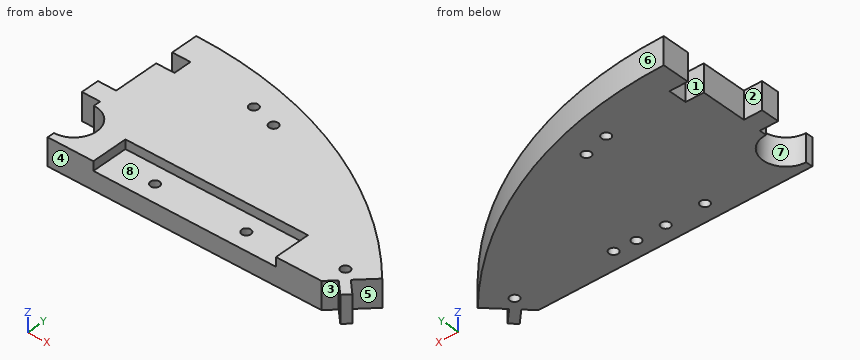
Autodesk Inventor part; units mm, degrees
ref_plane "YZ Plane" through (0, 0, 0) normal (1, 0, 0) x (0, 1, 0)
ref_plane "XZ Plane" through (0, 0, 0) normal (0, 1, 0) x (-1, 0, 0)
ref_plane "XY Plane" through (0, 0, 0) normal (0, 0, 1) x (1, 0, 0)
sketch "Sketch1" plane through (0, 0, 0) normal (0, 0, 1) x (1, 0, 0)
  circle A0 centre (0, -132.2876) radius 225 construction
  circle A1 centre (0, -132.2876) radius 200 construction
  line L0 (-225, -132.2876) -> (225, -132.2876) construction
  line L1 (150, -132.2876) -> (150, 35.4175) construction
  line L2 (175, -132.2876) -> (175, 9.1338) construction
  line L3 (0, 92.7124) -> (0, -357.2876) construction
  line L4 (150, 0) -> (0, 0)
  line L5 (0, 0) -> (0, 92.7124)
  line L6 (150, 0) -> (167.7086, 17.7086)
  line L7 (150, 0) -> (175.0437, 0) construction
  arc A2 (167.7086, 17.7086) -> (0, 92.7124) centre (0, -132.2876) ccw
  dimension "d0" = 450
  dimension "d1" = 25
  dimension "d2" = 75
  dimension "d3" = 25
  dimension "d4" = 45
extrude "Extrusion1" add sketch "Sketch1" along normal blind 15
sketch "Sketch2" plane through (0, 0, 15) normal (0, 0, 1) x (1, 0, 0)
  line L0 (10, 77.7124) -> (0, 77.7124)
  line L1 (0, 77.7124) -> (0, 67.7124)
  line L2 (0, 67.7124) -> (10, 67.7124)
  line L3 (10, 67.7124) -> (10, 77.7124)
  line L4 (0, 92.7124) -> (0, 0)
  line L5 (0, 0) -> (150, 0)
  line L6 (150, 0) -> (167.7086, 17.7086)
  arc A0 (167.7086, 17.7086) -> (0, 92.7124) centre (0, -132.2876) ccw
  line L7 (0, 92.7124) -> (0, 0)
  dimension "d7" = 10
  dimension "d8" = 10
  dimension "d21" = 15
extrude "Extrusion2" cut sketch "Sketch2" against normal blind 15 contours L3 L2 L1 L0
sketch "Sketch3" plane through (0, 0, 15) normal (0, 0, 1) x (1, 0, 0)
  line L0 (-10, 42.7124) -> (0, 42.7124)
  line L1 (0, 42.7124) -> (0, 32.7124)
  line L2 (0, 32.7124) -> (-10, 32.7124)
  line L3 (-10, 32.7124) -> (-10, 42.7124)
  line L4 (0, 0) -> (150, 0)
  line L5 (150, 0) -> (167.7086, 17.7086)
  arc A0 (167.7086, 17.7086) -> (0, 92.7124) centre (0, -132.2876) ccw
  line L6 (0, 67.7124) -> (0, 0)
  line L7 (0, 67.7124) -> (0, 0)
  line L8 (10, 67.7124) -> (0, 67.7124)
  line L9 (0, 92.7124) -> (0, 77.7124)
  line L10 (0, 77.7124) -> (10, 77.7124)
  line L11 (10, 77.7124) -> (10, 67.7124)
  dimension "d15" = 10
  dimension "d16" = 10
  dimension "d20" = 25
extrude "Extrusion3" add sketch "Sketch3" against normal blind 15 contours L0 L1 L2 L3
sketch "Sketch4" plane through (0, 0, 15) normal (0, 0, 1) x (1, 0, 0)
  line L0 (155, 5) -> (162.0711, -2.0711)
  line L1 (162.0711, -2.0711) -> (165.6066, 1.4645)
  line L2 (165.6066, 1.4645) -> (158.5355, 8.5355)
  line L3 (158.5355, 8.5355) -> (155, 5)
  line L4 (10, 67.7124) -> (0, 67.7124)
  line L5 (0, 67.7124) -> (0, 42.7124)
  line L6 (-10, 42.7124) -> (0, 42.7124)
  line L7 (-10, 32.7124) -> (-10, 42.7124)
  line L8 (0, 32.7124) -> (-10, 32.7124)
  line L9 (0, 32.7124) -> (0, 0)
  line L10 (0, 0) -> (150, 0)
  line L11 (150, 0) -> (167.7086, 17.7086)
  arc A0 (167.7086, 17.7086) -> (0, 92.7124) centre (0, -132.2876) ccw
  line L12 (0, 92.7124) -> (0, 77.7124)
  line L13 (0, 77.7124) -> (10, 77.7124)
  line L14 (10, 77.7124) -> (10, 67.7124)
  line L15 (150, 0) -> (167.7086, 17.7086)
  dimension "d22" = 10
  dimension "d23" = 5
  dimension "d24" = 5
extrude "Extrusion4" add sketch "Sketch4" against normal blind 15 contours L3 L2 L1 L0
sketch "Sketch5" plane through (0, 0, 15) normal (0, 0, 1) x (1, 0, 0)
  line L0 (10, 67.7124) -> (0, 67.7124) construction
  line L1 (0, 67.7124) -> (0, 42.7124) construction
  line L2 (-10, 42.7124) -> (0, 42.7124) construction
  line L3 (-10, 32.7124) -> (-10, 42.7124) construction
  line L4 (0, 32.7124) -> (-10, 32.7124) construction
  line L5 (0, 32.7124) -> (0, 0) construction
  line L6 (0, 0) -> (150, 0) construction
  line L7 (150, 0) -> (155, 5) construction
  line L8 (155, 5) -> (162.0711, -2.0711) construction
  line L9 (162.0711, -2.0711) -> (165.6066, 1.4645) construction
  line L10 (165.6066, 1.4645) -> (158.5355, 8.5355) construction
  line L11 (158.5355, 8.5355) -> (167.7086, 17.7086) construction
  arc A0 (167.7086, 17.7086) -> (0, 92.7124) centre (0, -132.2876) ccw construction
  line L12 (0, 92.7124) -> (0, 77.7124) construction
  line L13 (0, 77.7124) -> (10, 77.7124) construction
  line L14 (10, 77.7124) -> (10, 67.7124) construction
  circle A1 centre (0, -132.2876) radius 225 construction
  arc A2 (167.7086, 17.7086) -> (0, 92.7124) centre (0, -132.2876) ccw construction
  circle A3 centre (0, -132.2876) radius 210 construction
  circle A4 centre (50, 71.6732) radius 2.5
  circle A5 centre (64.4318, 67.5838) radius 2.5
  circle A6 centre (152.0028, 12.6094) radius 2.5
  dimension "d27" = 450
  dimension "d28" = 15
  dimension "d31" = 5
  dimension "d32" = 5
  dimension "d33" = 15
  dimension "d34" = 50
  dimension "d46" = 5
  dimension "d49" = 7.5
extrude "Extrusion5" cut sketch "Sketch5" against normal through all
thread "Thread1"
thread "Thread2"
thread "Thread4"
sketch "Sketch7" plane through (0, 0, 15) normal (0, 0, 1) x (1, 0, 0)
  line L0 (0, 0) -> (150, 0) construction
  line L1 (25, 0) -> (125, 0) construction
  line L2 (125, 0) -> (125, 20) construction
  line L3 (125, 20) -> (25, 20) construction
  line L4 (25, 20) -> (25, 0) construction
  circle A0 centre (50, 10) radius 2.5
  circle A1 centre (100, 10) radius 2.5
  dimension "d52" = 100
  dimension "d53" = 20
  dimension "d54" = 25
  dimension "d55" = 5
  dimension "d56" = 5
  dimension "d57" = 25
  dimension "d58" = 25
extrude "Extrusion6" cut sketch "Sketch7" against normal through all
thread "Thread5"
thread "Thread6"
sketch "Sketch8" plane through (0, 0, 15) normal (0, 0, 1) x (1, 0, 0)
  line L0 (0, 0) -> (150, 0)
  line L1 (25, 0) -> (125, 0)
  line L2 (125, 0) -> (125, 20)
  line L3 (125, 20) -> (25, 20)
  line L4 (25, 20) -> (25, 0)
  line L5 (0, 32.7124) -> (0, 0)
  dimension "d67" = 100
  dimension "d68" = 20
  dimension "d69" = 25
extrude "Extrusion7" cut sketch "Sketch8" against normal blind 5
sketch "Sketch9" plane through (0, 0, 15) normal (0, 0, 1) x (1, 0, 0)
  line L0 (0, 32.7124) -> (0, 0)
  circle A0 centre (0, 16.3562) radius 12.5
  dimension "d72" = 25
extrude "Extrusion8" cut sketch "Sketch9" against normal through all
sketch "Sketch10" plane through (0, 0, 0) normal (0, 0, -1) x (-1, 0, 0)
  circle A0 centre (-72, 9.4249) radius 2.5
  circle A1 centre (-88, 9.4249) radius 2.5
  point P0 (0, 0)
  dimension "d75" = 5
  dimension "d76" = 5
  dimension "d77" = 16
  dimension "d79" = 88
  dimension "d80" = 9.4249
extrude "Extrusion9" cut sketch "Sketch10" against normal blind 5
thread "Thread8"
thread "Thread9"
equation "\"d35\" = d46"
properties part number "CP006" material "ABS Plastic"
Read the model definition and answer for the solid it produces. Units are mm, in the model's axes. Face numbers are marked on the shaded views. A direction names the side the tool comes from. Coordinates: 2 decimals unless noted, no trailing zeros. Order: outer loops, then holes, each group sorted by start corner. A loop starts at its lowest first (then second) coordinate and runs counter-clockwise, first axis right, second up. Notation, with made-up numbers: (-8.5, 30) - (45.5, 30) arc R22 cw to (45.5, 43) - close; hole circle Ø8 at (8, -30.75). An arc over 180 degrees is marked (long way). Answer as a JSON object with one key per item and string values. Group by question number.
Item 1: Section B-B (x = 100) is taken. Give the vertices of the cut face in (y, z), plus the area to 3 significant figures.
Item 2: A tool of negligible diameter and unlimited length cuts with its end or side. For the marked faces 1, 2, 3, 4 and 5, from which of +Z, -Z, +X, -X, +Y, -Y can it reach the whole face along a straight path? Write none if from no direction.
Item 3: The mould has two halves that part along Y. Classify the marked faces 6, 7 and 8: +Y half, -Y half, draft (parallel to the pull), parting line (faces both ways), or undercut.
Item 4: Section A-A (z = 3) is taken. Give the vertices of the cut face in (x, y).
Item 5: Section C-C (z = 12) is taken. Give the vertices of the cut face in (x, y).
Item 6: Consider probe 1 along Z at (x, y) = (60.5, 7.5); probe 2 along Y at (x, z) = (100, 6.25); probe 3 along X at (y, z) = (30.5, 14). Determine where each line is inside the solid, lowest interval first. Write a range as from..to.
Item 7: Section D-D (x = 22.5) is taken. Give the vertices of the cut face in (y, z).
Item 8: Flat-ended cylindrical pins translate along their axes: P1, Ø8, axis at x = 4.5, z = 7, coming from the +Y side; P2, Ø2, axis at x = 120.5, z = 11.5, coming from the +Y side; P3, Ø3, axis at x = 4, z = 5.5, coming from the -Y side. Find the tip coordinate at first contact, or state that the pin passes through.
Results are:
{
 "1": {"outline": "(0, 0) - (7.5, 0) - (7.5, 10) - (0, 10) - close; (12.5, 0) - (69.27, 0) - (69.27, 15) - (20, 15) - (20, 10) - (12.5, 10) - close", "area": "889 mm^2"},
 "2": {"face 1": "+Z, -Z, -X", "face 2": "+Z, -Z, -X, +Y", "face 3": "+Z, -Z, -Y", "face 4": "+Z, -Z, -X, -Y", "face 5": "+Z, -Z, +X"},
 "3": {"face 6": "+Y half", "face 7": "undercut", "face 8": "draft"},
 "4": {"outline": "(-10, 32.71) - (0, 32.71) - (0, 28.86) arc R12.5 cw to (0, 3.86) - (0, 0) - (150, 0) - (155, 5) - (162.07, -2.07) - (165.61, 1.46) - (158.54, 8.54) - (167.71, 17.71) arc R225 ccw to (0, 92.71) - (0, 77.71) - (10, 77.71) - (10, 67.71) - (0, 67.71) - (0, 42.71) - (-10, 42.71) - close; hole circle Ø5 at (50, 10); hole circle Ø5 at (50, 71.67); hole circle Ø5 at (64.43, 67.58); hole circle Ø5 at (72, 9.42); hole circle Ø5 at (88, 9.42); hole circle Ø5 at (100, 10); hole circle Ø5 at (152, 12.61)"},
 "5": {"outline": "(-10, 32.71) - (0, 32.71) - (0, 28.86) arc R12.5 cw to (0, 3.86) - (0, 0) - (25, 0) - (25, 20) - (125, 20) - (125, 0) - (150, 0) - (155, 5) - (162.07, -2.07) - (165.61, 1.46) - (158.54, 8.54) - (167.71, 17.71) arc R225 ccw to (0, 92.71) - (0, 77.71) - (10, 77.71) - (10, 67.71) - (0, 67.71) - (0, 42.71) - (-10, 42.71) - close; hole circle Ø5 at (50, 71.67); hole circle Ø5 at (64.43, 67.58); hole circle Ø5 at (152, 12.61)"},
 "6": {"probe 1": "z = 0..10", "probe 2": "y = 0..7.5, 12.5..69.27", "probe 3": "x = 0..155.32"},
 "7": {"outline": "(0, 0) - (91.58, 0) - (91.58, 15) - (0, 15) - close"},
 "8": {"P1": "stops at y = 92.71", "P2": "stops at y = 58.36", "P3": "stops at y = 0"}
}
